Could you check a few things on this model? Use its own coordinates, in mm. A direction names the side the tool comes from. Coordinates: 2 decimals unless noted, no trailing zeros. Loops run counter-clockwise (first coordinate to the right, second up) from the corner with the lowest first, then second, coordinate; pieces in that order, holes last. Notation, with made-up numbers: (32, 28.25) -> (44, 28.25) arc R27 ccw to (44, 53.25) -> close; hole circle Ø8 at (-27, 43.5). An arc over 180 degrees is marked (long way). One line per question, with ' | ' between items.
from build123d import *

# Parameters (mm, degrees)
F1_DEPTH = 63.5
F2_DEPTH = 7.9375
F0_W     = 25.4
F0_H     = 19.05
F3_DEPTH = 25.4
F5_R     = 6.35


with BuildPart() as f1:
    # F0 (on Front) → F1 (new body, symmetric)
    with BuildSketch(Plane.XZ):
        Polygon((-41.275, 9.525), (-41.275, -9.525), (41.275, -9.525), (41.275, 9.525), (22.225, 9.525), align=None)
    extrude(amount=F1_DEPTH, both=True)

    # F0 (on Front) → F2 (join, symmetric)
    with BuildSketch(Plane.XZ):
        with BuildLine():
            add(Edge.make_bspline(
                [(-41.275, 9.525), (-40.5524685808, 30.7933831183), (10.8961521527, 58.542204844), (53.2054273143, 61.7017269308)],
                knots=[0, 0, 0, 0, 108.12000921, 108.12000921, 108.12000921, 108.12000921], degree=3))
            Line((-41.275, 9.525), (22.225, 9.525))
            Line((22.225, 9.525), (22.225, 27.0002))
            ThreePointArc((22.225, 27.0002), (31.096978812, 50.2595145208), (53.2054273143, 61.7017269308))
        make_face()
    extrude(amount=F2_DEPTH, both=True)

    # F0 (on Front) → F3 (join, symmetric)
    with BuildSketch(Plane.XZ):
        with Locations((73.025, 52.4002)):
            Rectangle(F0_W, F0_H)
        with BuildLine():
            Line((22.225, 9.525), (41.275, 9.525))
            Line((41.275, 9.525), (41.275, 27.0002))
            ThreePointArc((41.275, 27.0002), (45.9246798487, 38.2255201513), (57.15, 42.8752))
            Line((57.15, 42.8752), (60.325, 42.8752))
            Line((60.325, 42.8752), (60.325, 61.9252))
            Line((60.325, 61.9252), (57.15, 61.9252))
            add(Edge.make_bspline(
                [(53.2054273143, 61.7017269308), (54.5298526747, 61.8006308038), (55.8453223482, 61.8754395085), (57.15, 61.9252)],
                knots=[108.12000921, 108.12000921, 108.12000921, 108.12000921, 111.5045361635, 111.5045361635, 111.5045361635, 111.5045361635], degree=3))
            ThreePointArc((53.2054273143, 61.7017269308), (31.096978812, 50.2595145208), (22.225, 27.0002))
            Line((22.225, 27.0002), (22.225, 9.525))
        make_face()
    extrude(amount=F3_DEPTH, both=True)

    # F0 (on Front) → F4 (revolve)
    with BuildSketch(Plane.XZ):
        Polygon((85.725, 66.675), (85.725, 61.9252), (85.725, 42.8752), (85.725, 38.1), (111.125, 38.1), (111.125, 66.675), align=None)
    revolve(axis=Axis((85.725, 0, 52.3875), (0, 0, 1)))

    # F5
    f5_edges = [f1.edges().sort_by_distance(p)[0] for p in [
        (41.275, -63.5, 0),
        (-41.275, -63.5, 0),
        (41.275, 63.5, 0),
        (-41.275, 63.5, 0),
    ]]
    fillet(f5_edges, radius=F5_R)


solid = f1.part
1) If we section it at B-B on x = 94: Please give me the cut outline in (y, z) (3 decimals), and give its area (3 significant figures).
Data:
outline: (-24.014, 38.1) -> (24.014, 38.1) -> (24.014, 66.675) -> (-24.014, 66.675) -> close | area: 1,370 mm²
2) I'm going to push flat-ended pins straight in: pin 1 Ø4 at (x, y) = (42, -5) entering from +Z; pin 2 Ø8 at (y, z) = (-23.5, 32) entering from +X; pin 3 Ø15 at (x, y) = (89, 7.5) entering from -Z. Where does each tip first touch, or does it pass through?
Data:
pin 1: z = 60.66 | pin 2: x = 44.07 | pin 3: z = 38.1
3) If we section it at A-A on y = -52: Please give me the cut outline in (x, z) (3 decimals), and give its area (3 significant figures).
Data:
outline: (-41.275, -9.525) -> (41.275, -9.525) -> (41.275, 9.525) -> (-41.275, 9.525) -> close | area: 1,570 mm²
4) On a 3-axis mill with a long thin cutter (end or side, diameter ignored), from which of +Z, -Z, +X, -X, +Y, -Y can I reach the whole of each face in a straight line? I mean faces 1 (the face through (31.336, -16.791, 50.524)), 2 (the face through (86, 0, 38.1)), 3 (the face through (45.8, -0.4, 38.1)). Say none if no direction works.
Data:
face 1: +Z, -X, -Y | face 2: -Z, +X, +Y, -Y | face 3: -Z, +Y, -Y
5) I need wall thicknesses on line 1 along Y through (x, z) = (29, 50); line 2 along X through (y, z) = (12.5, 24) (3 decimals); line 3 along Y through (x, z) = (36.5, 47.5). Which ranges of each line are inside material? Lowest first, please. Write a range as from..to.
Data:
line 1: -7.94..7.94 | line 2: 22.225..41.275 | line 3: -25.4..25.4
